```python
from build123d import *

# Parameters (mm, degrees)
SKETCH2_W                                     = 300
SKETCH2_H                                     = 150
BOSS_EXTRUDE1_DEPTH                           = 120
CUT_EXTRUDE2_DEPTH                            = 5
CUT_EXTRUDE3_DEPTH                            = 110
CBORE_FOR_M4_PAN_HEAD_MACHINE_SCREW1_AT_COUNT = 2
CBORE_FOR_M4_PAN_HEAD_MACHINE_SCREW1_AT_PITCH = 256
CBORE_FOR_M4_PAN_HEAD_MACHINE_SCREW1_2_COUNT  = 2
CBORE_FOR_M4_PAN_HEAD_MACHINE_SCREW1_2_PITCH  = 277.077606457
CBORE_FOR_M4_PAN_HEAD_MACHINE_SCREW1_3_COUNT  = 2
CBORE_FOR_M4_PAN_HEAD_MACHINE_SCREW1_3_PITCH  = 106
CUT_EXTRUDE5_DEPTH                            = 332.700165812
SKETCH17_R                                    = 15
CUT_EXTRUDE6_DEPTH                            = 20
SKETCH3_R                                     = 15
CUT_EXTRUDE1_DEPTH                            = 50


with BuildPart() as part:
    # Sketch2 → Boss-Extrude1 (new body)
    with BuildSketch(Plane(origin=(0, 0, 0), x_dir=(1, 0, 0), z_dir=(0, 1, 0))):
        Rectangle(SKETCH2_W, SKETCH2_H)
    extrude(amount=BOSS_EXTRUDE1_DEPTH)

    # Sketch7 → Cut-Extrude2 (cut)
    with BuildSketch(Plane.XZ):
        with BuildLine():
            Line((-120, 65), (120, 65))
            ThreePointArc((120, 65), (134.142135624, 59.142135624), (140, 45))
            Line((140, 45), (140, -45))
            ThreePointArc((140, -45), (134.142135624, -59.142135624), (120, -65))
            Line((120, -65), (-120, -65))
            ThreePointArc((-120, -65), (-134.142135624, -59.142135624), (-140, -45))
            Line((-140, -45), (-140, 45))
            ThreePointArc((-140, 45), (-134.142135624, 59.142135624), (-120, 65))
        make_face()
    extrude(amount=-CUT_EXTRUDE2_DEPTH, mode=Mode.SUBTRACT)

    # Sketch8 → Cut-Extrude3 (cut)
    with BuildSketch(Plane.XZ.offset(-5)):
        with BuildLine():
            Line((-91.715728753, 60), (91.715728753, 60))
            ThreePointArc((91.715728753, 60), (122.32233047, 47.32233047), (135, 16.715728753))
            Line((135, 16.715728753), (135, -16.715728753))
            ThreePointArc((135, -16.715728753), (122.32233047, -47.32233047), (91.715728753, -60))
            Line((91.715728753, -60), (-91.715728753, -60))
            ThreePointArc((-91.715728753, -60), (-122.32233047, -47.32233047), (-135, -16.715728753))
            Line((-135, -16.715728753), (-135, 16.715728753))
            ThreePointArc((-135, 16.715728753), (-122.32233047, 47.32233047), (-91.715728753, 60))
        make_face()
    extrude(amount=-CUT_EXTRUDE3_DEPTH, mode=Mode.SUBTRACT)

    # Sketch14 → CBORE for M4 Pan Head Machine Screw1 (revolve, cut)
    with BuildSketch(Plane(origin=(128, 0, -53), x_dir=(0, 0, -1), z_dir=(1, 0, 0))):
        Polygon((0, 0), (0, 31.351936393), (2.25, 30), (2.25, 3.1), (4.5, 3.1), (4.5, 0.025), (4.525, 0), align=None)
    cbore_for_m4_pan_head_machine_screw1 = revolve(axis=Axis((128, -6.35, -53), (0, 1, 0)), mode=Mode.SUBTRACT)

    # CBORE for M4 Pan Head Machine Screw1 at: CBORE for M4 Pan Head Machine Screw1 ×2
    with Locations(*[(-i * CBORE_FOR_M4_PAN_HEAD_MACHINE_SCREW1_AT_PITCH, 0, 0) for i in range(1, CBORE_FOR_M4_PAN_HEAD_MACHINE_SCREW1_AT_COUNT)]):
        add(cbore_for_m4_pan_head_machine_screw1, mode=Mode.SUBTRACT)

    # CBORE for M4 Pan Head Machine Screw1 2: CBORE for M4 Pan Head Machine Screw1 ×2
    with Locations(*[Vector(-0.9239288705910962, 0, 0.38256429797912606) * (i * CBORE_FOR_M4_PAN_HEAD_MACHINE_SCREW1_2_PITCH) for i in range(1, CBORE_FOR_M4_PAN_HEAD_MACHINE_SCREW1_2_COUNT)]):
        add(cbore_for_m4_pan_head_machine_screw1, mode=Mode.SUBTRACT)

    # CBORE for M4 Pan Head Machine Screw1 3: CBORE for M4 Pan Head Machine Screw1 ×2
    with Locations(*[(0, 0, i * CBORE_FOR_M4_PAN_HEAD_MACHINE_SCREW1_3_PITCH) for i in range(1, CBORE_FOR_M4_PAN_HEAD_MACHINE_SCREW1_3_COUNT)]):
        add(cbore_for_m4_pan_head_machine_screw1, mode=Mode.SUBTRACT)

    # Sketch15 → Cut-Extrude5 (cut, through all)
    with BuildSketch(Plane(origin=(150, 0, 0), x_dir=(0, 0, -1), z_dir=(1, 0, 0))):
        Polygon((-42, 100), (-23.029720743, 23.02020202), (-15.487735621, 24.878787879), (-34, 100), align=None)
        Polygon((-29, 100), (-10.773994919, 26.04040404), (-3.232009797, 27.898989899), (-21, 100), align=None)
        Polygon((-16, 100), (1.481730904, 29.060606061), (9.023716027, 30.919191919), (-8, 100), align=None)
        Polygon((-3, 100), (13.737456728, 32.080808081), (21.27944185, 33.939393939), (5, 100), align=None)
        Polygon((10, 100), (25.993182552, 35.101010101), (33.535167674, 36.95959596), (18, 100), align=None)
        Polygon((23, 100), (38.248908375, 38.121212121), (45.790893498, 39.97979798), (31, 100), align=None)
    extrude(amount=-CUT_EXTRUDE5_DEPTH, mode=Mode.SUBTRACT)

    # Sketch17 → Cut-Extrude6 (cut)
    with BuildSketch(Plane(origin=(0, 0, -75), x_dir=(-1, 0, 0), z_dir=(0, 0, -1))):
        with Locations((0, 60)):
            Circle(SKETCH17_R)
    extrude(amount=-CUT_EXTRUDE6_DEPTH, mode=Mode.SUBTRACT)

    # Sketch3 → Cut-Extrude1 (cut)
    with BuildSketch(Plane(origin=(0, 120, 0), x_dir=(1, 0, 0), z_dir=(0, 1, 0))):
        with Locations(Location((-70, 0, 0), (0, 0, 270))):
            Circle(SKETCH3_R)
        with Locations(Location((70, 0, 0), (0, 0, 270))):
            Circle(SKETCH3_R)
    extrude(amount=-CUT_EXTRUDE1_DEPTH, mode=Mode.SUBTRACT)


solid = part.part
```
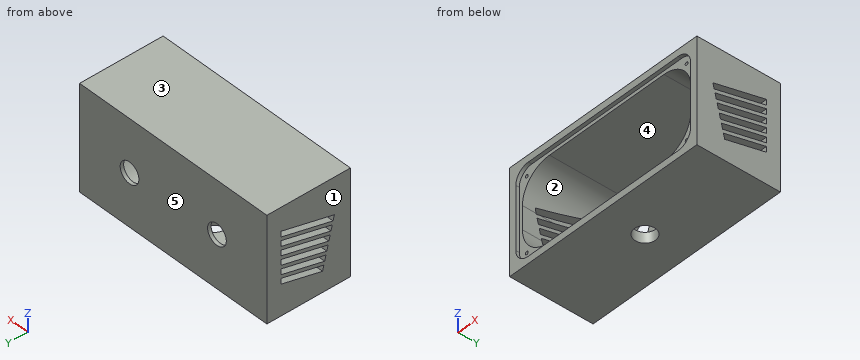
Build history of the part. All positions in model axes, mm. Face numbers are marked on the shaded views. A direction names the side the tool comes from. Give positions to 0.01 mm unless a question says otherwise; leave off trailing zeros. Order: outer loops, then holes, each group sorted by start corner. A loop starts at its lowest first (then second) coordinate and runs counter-clockwise, first axis right, second up. Notation, with made-up numbers: M 33.5,88 L 57.5,88 A19 cw 57.5,120 Z; hole C 38,8 d10. An arc over 180 degrees is marked long. Return JSON: item names as keys, results as strings.
Q1. Band-saw the part on B-B (y = 110.5). Give the cut face in (x, z).
Answer list:
{"outline": "M -150,-75 L 150,-75 L 150,75 L -150,75 Z; hole M -135,-16.72 A43.28 ccw -91.72,-60 L 91.72,-60 A43.28 ccw 135,-16.72 L 135,16.72 A43.28 ccw 91.72,60 L -91.72,60 A43.28 ccw -135,16.72 Z"}
Q2. Band-saw the part on A-A (x = 70). Give the cut face in (y, z).
Answer list:
{"outline": "M 0,-75 L 120,-75 L 120,-15 L 115,-15 L 115,-60 L 5,-60 L 5,-65 L 0,-65 Z; M 0,65 L 5,65 L 5,60 L 115,60 L 115,15 L 120,15 L 120,75 L 0,75 Z"}
Q3. Band-saw the part on C-C (x = 9). Give the cut face in (y, z), then the cut area to 3 significant figures.
Answer list:
{"outline": "M 0,-75 L 48,-75 L 48,-60 L 5,-60 L 5,-65 L 0,-65 Z; M 0,65 L 5,65 L 5,60 L 115,60 L 115,-60 L 72,-60 L 72,-75 L 120,-75 L 120,75 L 0,75 Z", "area": "3,790 mm^2"}
Q4. Flat gauge pins, fed straight in: pin 1 (3.5 mm diameter, centred on x = -128, z = 53, fed in from -Y); pin 2 (2.5 mm diameter, centred on x = -128, z = -53, fed in from -Y); pin 3 (1 mm diameter, centred on x = 52.5, z = -41.5, fed in from -Y). Where does each tip first touch, or does it go through?
Answer list:
{"pin 1": "stops at y = 30.3", "pin 2": "stops at y = 30.6", "pin 3": "stops at y = 115"}
Q5. Wall check: probe 1 along X at (y, z) = (117.65, 0); probe 2 along Z at (x, y) = (128, 24); probe 3 along X at (y, z) = (16.5, 53). Give the ranges that are in metal, low to high. Write a range as from..to.
Answer list:
{"probe 1": "x = -150..-85, -55..55, 85..150", "probe 2": "z = -75..-55.25, -50.75..-40.32, 40.32..50.75, 55.25..75", "probe 3": "x = -150..-130.25, -125.75..-115.32, 115.32..125.75, 130.25..150"}
Q6. Two-plate mould, pull along X, no slides. Class the marked faces 1, 2 and 3: pulls with the +X half, pulls with the -X half, needs draft (parallel to the pull), parting line crosses it, or undercut.
Answer list:
{"face 1": "pulls with the -X half", "face 2": "undercut", "face 3": "needs draft"}
Q7. 3-axis set-ups, long thin cutter, end or side, ignore diameter. For the marked faces 4 and 5: which of +Z, -Z, +X, -X, +Y, -Y reach the whole face in a straight line?
Answer list:
{"face 4": "-Y", "face 5": "+Z, -Z, +X, -X, +Y"}
Q8. Band-saw the part on D-D (y = 60). Count the separate pieces of the cut face and the enclosed holes in it, then the cut area to 3 significant figures.
Answer list:
{"separate pieces": "13", "enclosed holes": "0", "area": "12,200 mm^2"}
